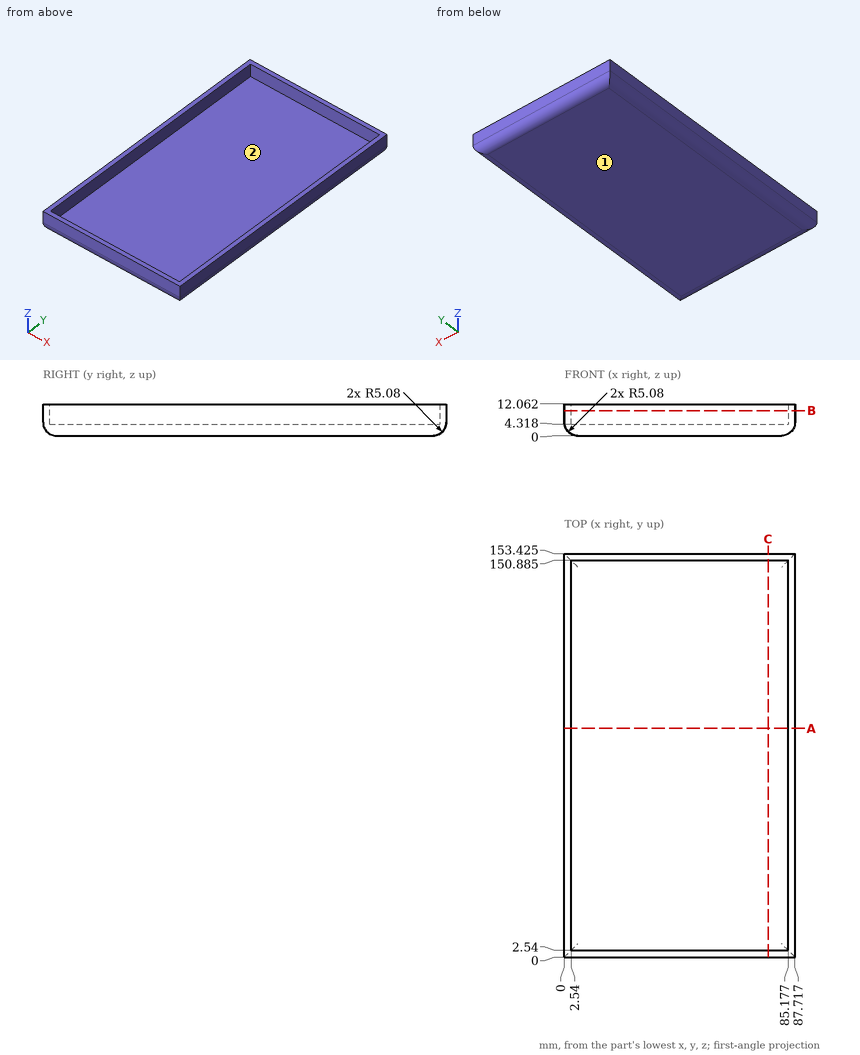
Verification items for this drawing (mm, ordinates from the low corner). Round coordinates to 2 decimals unless told otherwise and drop trailing zeros. Order: outer loops, then holes, each group sorted by start corner. A loop starts at its lowest first (then second) coordinate and runs counter-clockwise, first axis right, second up. Notation, with made-up numbers: (81.25, 14.5) -> (105.25, 14.5) arc R31 cw to (105.25, 49.5) -> close; hole circle Ø1 at (-31, 18.25). An arc over 180 degrees is marked (long way). Use one line per item in the form item = value.
1. Cross-section at B-B, the plane z = 9.5. Enter the section's corners in (x, y) (1 decimal), plus the area to 3 significant figures.
Working result:
outline = (0, 0) -> (87.7, 0) -> (87.7, 153.4) -> (0, 153.4) -> close; hole (2.5, 2.5) -> (85.2, 2.5) -> (85.2, 150.9) -> (2.5, 150.9) -> close
area = 1,200 mm^2
2. Cross-section at A-A, the plane y = 87. Enter the section's corners in (x, z).
Working result:
outline = (0, 5.08) arc R5.08 ccw to (5.08, 0) -> (82.64, 0) arc R5.08 ccw to (87.72, 5.08) -> (87.72, 12.06) -> (85.18, 12.06) -> (85.18, 4.32) -> (2.54, 4.32) -> (2.54, 12.06) -> (0, 12.06) -> close
3. Scan lines: line 1 along X through (y, z) = (77, 5.5); line 2 along Y through (x, z) = (50, 6.5) (1 decimal); line 3 along Z through (x, y) = (73.5, 30.5). Record each from-to range of solid material in increasing order. Write a range as from..to.
Working result:
line_1 = 0..2.54, 85.18..87.72
line_2 = 0..2.5, 150.9..153.4
line_3 = 0..4.32
4. Mould release check, pull along Y, two halves, no side actions. Record for the marked faces 1 and 2: pulls with the +Y half, pulls with the -Y half, needs draft (parallel to the pull), parting line crosses it, or undercut.
Working result:
face_1 = needs draft
face_2 = undercut
5. Go/stop test with flat-tipped pins: pin 1 (10 mm diameter, centred on x = 14, y = 125.5, fed in from +Z); pin 2 (2.5 mm diameter, centred on y = 67.5, z = 8, fed in from -X); pin 3 (1 mm diameter, centred on y = 59.5, z = 2.5, fed in from +X). Record where each tip stops, or that it passes through.
Working result:
pin_1 = 4.32
pin_2 = 0
pin_3 = 87.27
6. Cross-section at C-C, the plane x = 77.5. Enter the section's corners in (y, z) (1 decimal).
Working result:
outline = (0, 5.1) arc R5.1 ccw to (5.1, 0) -> (148.3, 0) arc R5.1 ccw to (153.4, 5.1) -> (153.4, 12.1) -> (150.9, 12.1) -> (150.9, 4.3) -> (2.5, 4.3) -> (2.5, 12.1) -> (0, 12.1) -> close
